For this review, take the finished solid that the model builds, in its own axes (mm). Face numbers are marked on the shaded views. A direction names the side the tool comes from. Round coordinates to 2 decimals unless told otherwise and drop trailing zeros. Order: outer loops, then holes, each group sorted by start corner. A loop starts at its lowest first (then second) coordinate and runs counter-clockwise, first axis right, second up. Notation, with made-up numbers: (-33, -24.75) -> (-28, -24.75) arc R30 ccw to (-28, -1.75) -> close; hole circle Ø9 at (64, 27.5). An arc over 180 degrees is marked (long way). Put each result on its own line as item: value. Start each with the question number.
```python
from build123d import *

# Parameters (mm, degrees)
SKETCH_2_W      = 78.232
SKETCH_2_H      = 75.184
SKETCH_2_R      = 1.5
EXTRUDE_1_DEPTH = 2
SKETCH_4_W      = 60.289914042
SKETCH_4_H      = 29.214557113
EXTRUDE_2_DEPTH = 10
SKETCH_5_W      = 9.086617177
SKETCH_5_H      = 2.41728743
EXTRUDE_3_DEPTH = 4
SKETCH_6_W      = 0.859863671
SKETCH_6_H      = 1.050944487
SKETCH_6_W_2    = 1.433106119
SKETCH_6_H_2    = 1.003174283
SKETCH_6_W_3    = 1.050944487
SKETCH_6_W_4    = 1.003174283
SKETCH_6_W_5    = 0.983317738
EXTRUDE_4_DEPTH = 10


with BuildPart() as part:
    # 草图2 → 凸台-拉伸1 (new body)
    with BuildSketch(Plane(origin=(0, 0, 0), x_dir=(1, 0, 0), z_dir=(0, 1, 0))):
        Rectangle(SKETCH_2_W, SKETCH_2_H)
        with Locations((35, -35)):
            Circle(SKETCH_2_R, mode=Mode.SUBTRACT)
        with Locations((35, 35)):
            Circle(SKETCH_2_R, mode=Mode.SUBTRACT)
        with Locations((-35, 35)):
            Circle(SKETCH_2_R, mode=Mode.SUBTRACT)
        with Locations((-35, -35)):
            Circle(SKETCH_2_R, mode=Mode.SUBTRACT)
    extrude(amount=EXTRUDE_1_DEPTH)

    # 草图4 → 凸台-拉伸2 (add)
    with BuildSketch(Plane(origin=(0, 2, 0), x_dir=(1, 0, 0), z_dir=(0, 1, 0))):
        with Locations((-0.127049012, 2.027434591)):
            Rectangle(SKETCH_4_W, SKETCH_4_H)
    extrude(amount=EXTRUDE_2_DEPTH)

    # 草图5 → 凸台-拉伸3 (add)
    with BuildSketch(Plane.ZY.offset(30.272006033)):
        with Locations((-6.851231395, 8.39841401)):
            Rectangle(SKETCH_5_W, SKETCH_5_H)
    extrude(amount=EXTRUDE_3_DEPTH)

    # 草图6 → 凸台-拉伸4 (add)
    with BuildSketch(Plane.ZY.offset(34.272006033)):
        with Locations((-8.824134234, 8.322199757)):
            Rectangle(SKETCH_6_W, SKETCH_6_H)
        with Locations((-7.199947299, 8.346084859)):
            Rectangle(SKETCH_6_W_2, SKETCH_6_H_2)
        with Locations((-5.384679549, 8.346084859)):
            Rectangle(SKETCH_6_W_3, SKETCH_6_H_2)
        with Locations((-3.784377716, 8.346084859)):
            Rectangle(SKETCH_6_W_4, SKETCH_6_H_2)
        with Locations((-10.446641143, 8.322199757)):
            Rectangle(SKETCH_6_W_5, SKETCH_6_H)
    extrude(amount=EXTRUDE_4_DEPTH)


solid = part.part
```
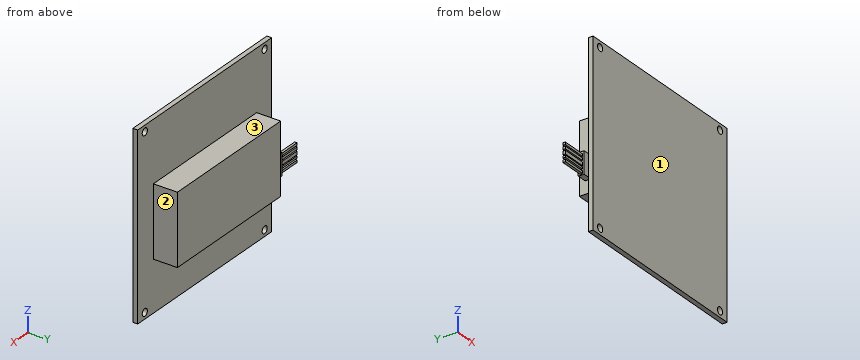
Item 1: Consider section D-D, the plane x = 14.5. Write out the cut boundary in (y, z), plus the area to 3 significant figures.
Item 2: Consider section C-C, the plane y = 1. Write out the cut boundary in (x, z).
Item 3: Insertion check: pin 1 Ø1.5 at (x, y) = (-24, 10.5) entering from +Z; pin 2 Ø5 at (y, z) = (9.5, -0.5) entering from -X; pin 3 Ø1.1 at (x, y) = (-38.5, 8.5) entering from -Z. Each pin has a flat end and moves straight along its axis. Give the tip position at first contact, or say it passes through.
Item 4: Consider section B-B, the plane x = 35. Write out the cut boundary in (y, z), plus the area to 3 significant figures.
Item 5: Tool access review of the marked faces 1, 2 and 3: name each direction out of +Z, -Z, +X, -X, +Y, -Y from which nothing blocks a thin tool from reaching the whole face with its end or side.
Item 6: For L1, parallel to X at y = 0.8, z = -35; L2, parallel to Z at x = 35, y = 1.6; L3, parallel to Z at x = 20, y = 2.25, list the stretches that pass through material, from the lowest coordinate up.
Item 7: Consider section A-A, the plane z = -35. Write out the cut boundary in (x, y), plus the area to 3 significant figures.
Evaluation:
1. outline: (0, -37.59) -> (2, -37.59) -> (2, -16.63) -> (12, -16.63) -> (12, 12.58) -> (2, 12.58) -> (2, 37.59) -> (0, 37.59) -> close
1. area: 443 mm^2
2. outline: (-39.12, -37.59) -> (39.12, -37.59) -> (39.12, 37.59) -> (-39.12, 37.59) -> close; hole circle Ø3 at (-35, -35); hole circle Ø3 at (-35, 35); hole circle Ø3 at (35, -35); hole circle Ø3 at (35, 35)
3. pin 1: stops at z = 12.58
3. pin 2: stops at x = -34.27
3. pin 3: stops at z = -10.94
4. outline: (0, -37.59) -> (2, -37.59) -> (2, -36.5) -> (0, -36.5) -> close; (0, -33.5) -> (2, -33.5) -> (2, 33.5) -> (0, 33.5) -> close; (0, 36.5) -> (2, 36.5) -> (2, 37.59) -> (0, 37.59) -> close
4. area: 138 mm^2
5. face 1: +Z, -Z, +X, -X, -Y
5. face 2: +Z, -Z, +X, +Y
5. face 3: +Z, +X, -X, +Y
6. L1: x = -39.12 to -36.5, -33.5 to 33.5, 36.5 to 39.12
6. L2: z = -37.59 to -36.5, -33.5 to 33.5, 36.5 to 37.59
6. L3: z = -16.63 to 12.58
7. outline: (-39.12, 0) -> (-36.5, 0) -> (-36.5, 2) -> (-39.12, 2) -> close; (-33.5, 0) -> (33.5, 0) -> (33.5, 2) -> (-33.5, 2) -> close; (36.5, 0) -> (39.12, 0) -> (39.12, 2) -> (36.5, 2) -> close
7. area: 144 mm^2
